```python
from build123d import *

# Parameters (mm, degrees)
F0_W     = 130
F0_H     = 120
F1_DEPTH = 50
F4_R     = 42.5
F5_DEPTH = 100


with BuildPart() as f1:
    # F0 (on Top) → F1 (new body)
    with BuildSketch(Plane.XY):
        with Locations((-1.133092, -1.057171)):
            Rectangle(F0_W, F0_H)
    extrude(amount=F1_DEPTH)

    # F2: F1 across face


with BuildPart() as f1_1:
    add(f1.part)
    add(f1.part.mirror(Plane(origin=(-1.133092, -1.057171, 0), x_dir=(1, 0, 0), z_dir=(0, 0, -1))))

    # F4 (on face) → F5 (cut)
    with BuildSketch(Plane.XY.offset(50)):
        Circle(F4_R)
    extrude(amount=-F5_DEPTH, mode=Mode.SUBTRACT)


solid = f1_1.part
```
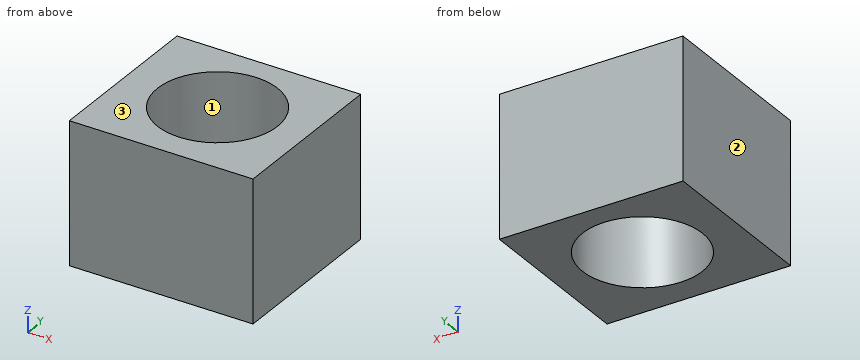
Model file for the job. Use its own axes, mm. Face numbers are marked on the shaded views. Coordinates: 2 decimals unless noted, no trailing zeros. Order: outer loops, then holes, each group sorted by start corner. A loop starts at its lowest first (then second) coordinate and runs counter-clockwise, first axis right, second up. Notation, with made-up numbers: (60.5, 13) -> (105.5, 13) arc R24 cw to (105.5, 47) -> close; hole circle Ø5 at (55.5, -6.5). An arc over 180 degrees is marked (long way). Answer as a JSON object with one key per item and string values. Group by question number.
1) Cut at C-C, the plane y = 0. Write the cut outline in (x, z), then the cut area to 3 significant figures.
2) Cut at B-B, the plane z = -7. Write the cut outline in (x, y), then the cut area to 3 significant figures.
3) Pull direction X, two halves, no side cores. Call the marked faces 1, 2 and 3: +X half, -X half, draft (parallel to the pull), parting line (faces both ways), or undercut.
4) Drill centre lines: L1, parallel to Y at x = 0, z = 4; L2, parallel to X at y = -35, z = 34.5; L3, parallel to X at y = -28, z = -38.5. Where is each one in solid material? Low to high.
5) Cut at A-A, the plane x = 0. Write the cut outline in (y, z), then the cut area to 3 significant figures.
Check values:
{
 "1": {"outline": "(-66.13, -50) -> (-42.5, -50) -> (-42.5, 50) -> (-66.13, 50) -> close; (42.5, -50) -> (63.87, -50) -> (63.87, 50) -> (42.5, 50) -> close", "area": "4,500 mm²"},
 "2": {"outline": "(-66.13, -61.06) -> (63.87, -61.06) -> (63.87, 58.94) -> (-66.13, 58.94) -> close; hole circle Ø85 at (0, 0)", "area": "9,930 mm²"},
 "3": {"face 1": "undercut", "face 2": "-X half", "face 3": "draft"},
 "4": {"L1": "y = -61.06 to -42.5, 42.5 to 58.94", "L2": "x = -66.13 to -24.11, 24.11 to 63.87", "L3": "x = -66.13 to -31.97, 31.97 to 63.87"},
 "5": {"outline": "(-61.06, -50) -> (-42.5, -50) -> (-42.5, 50) -> (-61.06, 50) -> close; (42.5, -50) -> (58.94, -50) -> (58.94, 50) -> (42.5, 50) -> close", "area": "3,500 mm²"}
}
